from build123d import *

# Parameters (mm, degrees)
SKETCH1_W                = 48
SKETCH1_H                = 38
BOSS_EXTRUDE1_DEPTH      = 2
SKETCH2_W                = 44
SKETCH2_H                = 36
BOSS_EXTRUDE2_DEPTH      = 2
SKETCH3_W                = 4
SKETCH3_H                = 30
BOSS_EXTRUDE3_DEPTH      = 2
CHAMFER1_SIZE            = 1
BOSS_EXTRUDE4_DEPTH      = 12
FILLET1_R                = 0.5
SKETCH5_W                = 1
SKETCH5_H                = 26
BOSS_EXTRUDE5_DEPTH      = 8.5
CHAMFER2_SIZE            = 0.5
CHAMFER2_OF_MIRROR1_SIZE = 0.5
SKETCH6_W                = 10
SKETCH6_H                = 1
BOSS_EXTRUDE6_DEPTH      = 2
FILLET2_R                = 1
SKETCH7_W                = 0.95
SKETCH7_H                = 1.9
SKETCH7_H_2              = 11.2
BOSS_EXTRUDE7_DEPTH      = 4.5
SKETCH8_W                = 1.9
SKETCH8_H                = 11.2
BOSS_EXTRUDE8_DEPTH      = 4
SKETCH9_W                = 1
SKETCH9_H                = 6.5
BOSS_EXTRUDE9_DEPTH      = 9
FILLET3_R                = 1
SKETCH10_R               = 0.75
CUT_EXTRUDE1_DEPTH       = 2
FILLET3_OF_MIRROR2_R     = 1
CUT_EXTRUDE2_DEPTH       = 2
FILLET4_R                = 1
FILLET5_R                = 2


with BuildPart() as part:
    # Sketch1 → Boss-Extrude1 (new body)
    with BuildSketch(Plane(origin=(0, 0, 0), x_dir=(1, 0, 0), z_dir=(0, 1, 0))):
        Rectangle(SKETCH1_W, SKETCH1_H)
    extrude(amount=BOSS_EXTRUDE1_DEPTH)

    # Sketch2 → Boss-Extrude2 (add)
    with BuildSketch(Plane(origin=(0, 2, 0), x_dir=(1, 0, 0), z_dir=(0, 1, 0))):
        with Locations((0, -1)):
            Rectangle(SKETCH2_W, SKETCH2_H)
    extrude(amount=BOSS_EXTRUDE2_DEPTH)

    # Sketch3 → Boss-Extrude3 (add)
    with BuildSketch(Plane(origin=(0, 4, 0), x_dir=(1, 0, 0), z_dir=(0, 1, 0))):
        with Locations((-19.5, -4)):
            Rectangle(SKETCH3_W, SKETCH3_H)
        with Locations((19.5, -4)):
            Rectangle(SKETCH3_W, SKETCH3_H)
    extrude(amount=BOSS_EXTRUDE3_DEPTH)

    # Chamfer1
    chamfer1_edges = [part.edges().sort_by_distance(p)[0] for p in [
        (-21.5, 5, 19),
        (-17.5, 5, 19),
        (17.5, 5, 19),
        (21.5, 5, 19),
    ]]
    chamfer(chamfer1_edges, length=CHAMFER1_SIZE)

    # Sketch4 → Boss-Extrude4 (add)
    with BuildSketch(Plane(origin=(0, 4, 0), x_dir=(1, 0, 0), z_dir=(0, 1, 0))):
        Polygon((22, 17), (-22, 17), (-22, 11), (-21.5, 11), (-17.5, 11), (-17.5, 12.5), (17.5, 12.5), (17.5, 11), (21.5, 11), (22, 11), align=None)
    extrude(amount=BOSS_EXTRUDE4_DEPTH)

    # Fillet1
    fillet1_edges = [part.edges().sort_by_distance(p)[0] for p in [
        (17.5, 11, -11),
        (17.5, 16, -11.75),
        (22, 10, -11),
        (-22, 10, -11),
        (-17.5, 11, -11),
        (19.75, 16, -11),
        (22, 16, -14),
        (0, 16, -17),
        (-22, 16, -14),
        (-19.75, 16, -11),
        (-17.5, 16, -11.75),
        (0, 16, -12.5),
        (-22, 9, -17),
        (22, 9, -17),
    ]]
    fillet(fillet1_edges, radius=FILLET1_R - 0.0001)  # a hair under: the kernel refuses the full size

    # Sketch5 → Boss-Extrude5 (add)
    with BuildSketch(Plane(origin=(0, 6, 0), x_dir=(1, 0, 0), z_dir=(0, 1, 0))):
        with Locations((-19.5, -2)):
            Rectangle(SKETCH5_W, SKETCH5_H)
    boss_extrude5 = extrude(amount=BOSS_EXTRUDE5_DEPTH)

    # Chamfer2
    chamfer2_edges = [part.edges().sort_by_distance(p)[0] for p in [
        (-19, 10.25, 15),
        (-20, 10.25, 15),
    ]]
    chamfer(chamfer2_edges, length=CHAMFER2_SIZE - 0.0001)  # a hair under: the kernel refuses the full size

    # Mirror1: Boss-Extrude5 across plane
    add(boss_extrude5.mirror(Plane.ZY))

    # Chamfer2 of Mirror1
    chamfer2_of_mirror1_edges = [part.edges().sort_by_distance(p)[0] for p in [
        (19, 10.25, 15),
        (20, 10.25, 15),
    ]]
    chamfer(chamfer2_of_mirror1_edges, length=CHAMFER2_OF_MIRROR1_SIZE - 0.0001)  # a hair under: the kernel refuses the full size

    # Sketch6 → Boss-Extrude6 (add)
    with BuildSketch(Plane.XZ):
        with Locations((0, 19.5)):
            Rectangle(SKETCH6_W, SKETCH6_H)
    extrude(amount=-BOSS_EXTRUDE6_DEPTH)

    # Fillet2
    fillet2_edges = [part.edges().sort_by_distance(p)[0] for p in [
        (-5, 1, 20),
        (5, 1, 20),
    ]]
    fillet(fillet2_edges, radius=FILLET2_R - 0.0001)  # a hair under: the kernel refuses the full size

    # Sketch7 → Boss-Extrude7 (add)
    with BuildSketch(Plane.XZ):
        Polygon((-10, -14), (-0.95, -14), (-0.95, -12.1), (-8.1, -12.1), (-8.1, -0.9), (-0.95, -0.9), (-0.95, 1), (-10, 1), align=None)
        with Locations((-0.475, -13.05)):
            Rectangle(SKETCH7_W, SKETCH7_H)
        with Locations((0.475, -13.05)):
            Rectangle(SKETCH7_W, SKETCH7_H)
        Polygon((0.95, -14), (10, -14), (10, 1), (0.95, 1), (0.95, -0.9), (8.1, -0.9), (8.1, -12.1), (0.95, -12.1), align=None)
        with Locations((-0.475, -6.5)):
            Rectangle(SKETCH7_W, SKETCH7_H_2)
        with Locations((0.475, -6.5)):
            Rectangle(SKETCH7_W, SKETCH7_H_2)
        with Locations((-0.475, 0.05)):
            Rectangle(SKETCH7_W, SKETCH7_H)
        with Locations((0.475, 0.05)):
            Rectangle(SKETCH7_W, SKETCH7_H)
    extrude(amount=BOSS_EXTRUDE7_DEPTH)

    # Sketch8 → Boss-Extrude8 (add)
    with BuildSketch(Plane.XZ.offset(4.5)):
        with Locations((0, -6.5)):
            Rectangle(SKETCH8_W, SKETCH8_H)
    extrude(amount=BOSS_EXTRUDE8_DEPTH)

    # Sketch9 → Boss-Extrude9 (add)
    with BuildSketch(Plane.XZ):
        with Locations((-4.525, -6.5)):
            Rectangle(SKETCH9_W, SKETCH9_H)
    boss_extrude9 = extrude(amount=BOSS_EXTRUDE9_DEPTH)

    # Fillet3
    fillet3_edges = [part.edges().sort_by_distance(p)[0] for p in [
        (-4.525, -9, -3.25),
        (-4.525, -9, -9.75),
    ]]
    fillet(fillet3_edges, radius=FILLET3_R)

    # Sketch10 → Cut-Extrude1 (cut)
    with BuildSketch(Plane.ZY.offset(5.025)):
        with Locations((-6.5, -6)):
            Circle(SKETCH10_R)
    cut_extrude1 = extrude(amount=-CUT_EXTRUDE1_DEPTH, mode=Mode.SUBTRACT)

    # Mirror2: Boss-Extrude9, Cut-Extrude1 across plane
    add(boss_extrude9.mirror(Plane.ZY))
    add(cut_extrude1.mirror(Plane.ZY), mode=Mode.SUBTRACT)

    # Fillet3 of Mirror2
    fillet3_of_mirror2_edges = [part.edges().sort_by_distance(p)[0] for p in [
        (4.525, -9, -3.25),
        (4.525, -9, -9.75),
    ]]
    fillet(fillet3_of_mirror2_edges, radius=FILLET3_OF_MIRROR2_R)

    # Sketch11 → Cut-Extrude2 (cut)
    with BuildSketch(Plane.XZ):
        Polygon((20, -11.4), (10, -11.4), (10, -14), (-10, -14), (-10, -11.4), (-20, -11.4), (-20, -15.2), (20, -15.2), align=None)
        Polygon((10, -1.9), (20, -1.9), (20, 17.1), (-20, 17.1), (-20, -1.9), (-10, -1.9), (-10, 1), (10, 1), align=None)
    extrude(amount=-CUT_EXTRUDE2_DEPTH, mode=Mode.SUBTRACT)

    # Fillet4
    fillet4_edges = [part.edges().sort_by_distance(p)[0] for p in [
        (0, -8.5, -12.1),
        (0, -8.5, -0.9),
    ]]
    fillet(fillet4_edges, radius=FILLET4_R)

    # Fillet5
    fillet5_edges = [part.edges().sort_by_distance(p)[0] for p in [
        (-24, 1, -19),
        (-24, 1, 19),
        (24, 1, 19),
        (24, 1, -19),
    ]]
    fillet(fillet5_edges, radius=FILLET5_R)


solid = part.part
The listing builds one solid part. Answer for the finished solid, in the listing's coordinates (mm). A direction names the side the tool comes from. Coordinates: 2 decimals unless noted, no trailing zeros. Write each loop counter-clockwise with the first axis right and the second up, starting at its lowest first coordinate (ties: lowest second). Pieces come first, ordered by that corner, then holes. Notation, with made-up numbers: (75.25, 63.25) - (112.25, 63.25) arc R14 cw to (112.25, 84.25) - close; hole circle Ø2 at (-35.5, -21.5). An arc over 180 degrees is marked (long way). Return JSON: item names as keys, results as strings.
1. Consider line 1 along X through (y, z) = (-5.25, -4) (3 decimals); line 2 along X through (y, z) = (0.5, 16); line 3 along X through (y, z) = (7, -5). Determine where each line is inside the solid, lowest interval first.
Final values:
{"line 1": "-5.025 to -4.025, -0.95 to 0.95, 4.025 to 5.025", "line 2": "-24 to -20, 20 to 24", "line 3": "-20 to -19, 19 to 20"}
2. The part is cut by section C-C on x = -12.5. Determine the outline of the cut face in (y, z), then the cut area to 3 significant figures.
Final values:
{"outline": "(0, -19) - (2, -19) - (2, -17) - (15.5, -17) arc R0.5 ccw to (16, -16.5) - (16, -13) arc R0.5 ccw to (15.5, -12.5) - (4, -12.5) - (4, 19) - (0, 19) - (0, 17.1) - (2, 17.1) - (2, -1.9) - (0, -1.9) - (0, -11.4) - (2, -11.4) - (2, -15.2) - (0, -15.2) - close", "area": "156 mm^2"}
3. The part is cut by section B-B on y = -6. Determine the outline of the cut face in (x, z) (3 decimals), then the cut area to 3 significant figures.
Final values:
{"outline": "(-5.025, -9.75) - (-4.025, -9.75) - (-4.025, -7.25) - (-5.025, -7.25) - close; (-5.025, -5.75) - (-4.025, -5.75) - (-4.025, -3.25) - (-5.025, -3.25) - close; (-0.95, -12.1) - (0.95, -12.1) - (0.95, -0.9) - (-0.95, -0.9) - close; (4.025, -9.75) - (5.025, -9.75) - (5.025, -7.25) - (4.025, -7.25) - close; (4.025, -5.75) - (5.025, -5.75) - (5.025, -3.25) - (4.025, -3.25) - close", "area": "31.3 mm^2"}
4. The part is cut by section A-A on y = -2.25. Determine the outline of the cut face in (x, z) (3 decimals).
Final values:
{"outline": "(-10, -14) - (10, -14) - (10, 1) - (-10, 1) - close; (-5.025, -9.75) - (-4.025, -9.75) - (-4.025, -3.25) - (-5.025, -3.25) - close; (4.025, -9.75) - (5.025, -9.75) - (5.025, -3.25) - (4.025, -3.25) - close; hole (-8.1, -12.1) - (-0.95, -12.1) - (-0.95, -0.9) - (-8.1, -0.9) - close; hole (0.95, -12.1) - (8.1, -12.1) - (8.1, -0.9) - (0.95, -0.9) - close"}
5. Each of these flat-tipped pins is pushed along its axis until it touches: pin 1 Ø1.2 at (x, z) = (19, 3.5) entering from +Y; pin 2 Ø12 at (x, y) = (-10.5, 6.5) entering from -Z; pin 3 Ø5 at (x, y) = (9, 4) entering from +Z; pin 4 Ø8 at (x, z) = (0.5, -1) entering from +Y. Where does it stop, or does it pass through?
Final values:
{"pin 1": "y = 14.5", "pin 2": "z = -19", "pin 3": "z = 19", "pin 4": "y = 4"}
6. For a pull along Z with two mould halves and no side action, classify faces 6 (the face through (0, 10, -12.5)), 7 (the face through (4.025, -4, -7)), 8 (the face through (0, -8.5, -6)) as +Z half, -Z half, draft (parallel to the pull), parting line (faces both ways), or undercut.
Final values:
{"face 6": "+Z half", "face 7": "undercut", "face 8": "draft"}
7. Which of the six approach directions +Z, -Z, +X, -X, +Y, -Y give full straight-line access (tool end or side, diameter ignored) to faces 1 (the face through (-19, 10, 2)), 2 (the face through (15, 1, -1.9)), 3 (the face through (21.8, 4, 4.8)), 4 (the face through (-23.4, 1.01, 18.43)), 5 (the face through (-21.5, 5, 4))?
Final values:
{"face 1": "+Z, +Y", "face 2": "-Y", "face 3": "+Z, +X, +Y", "face 4": "+Z, -X, +Y, -Y", "face 5": "+Z, -X, +Y"}
